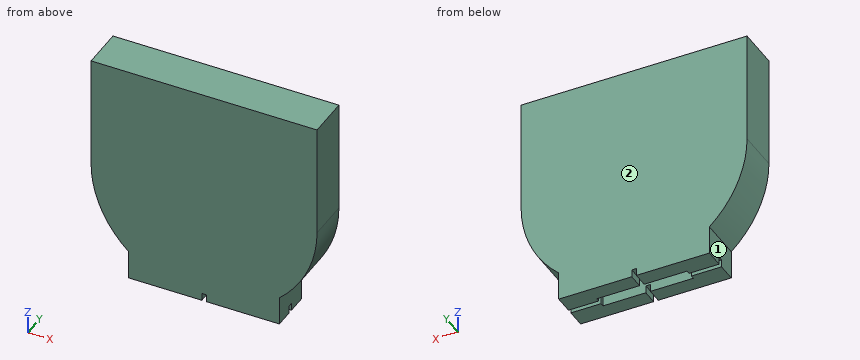
```python
from build123d import *

# Parameters (mm, degrees)
BOSS_EXTRUDE1_DEPTH = 0.8
BOSS_EXTRUDE2_DEPTH = 1
BOSS_EXTRUDE3_START = 1
BOSS_EXTRUDE3_DEPTH = 1
CUT_EXTRUDE1_DEPTH  = 0.5


with BuildPart() as part:
    # Sketch1 → Boss-Extrude1 (new body)
    with BuildSketch(Plane(origin=(0, 0, 0), x_dir=(1, 0, 0), z_dir=(0, 1, 0))):
        with BuildLine():
            Line((-5, 7.5), (-5, 5.590169944))
            ThreePointArc((-5, 5.590169944), (-6.846531969, 3.061862178), (-7.5, 0))
            Line((-7.5, 0), (-7.5, -7.5))
            Line((-7.5, -7.5), (7.5, -7.5))
            Line((7.5, -7.5), (7.5, 0))
            ThreePointArc((7.5, 0), (6.846531969, 3.061862178), (5, 5.590169944))
            Line((5, 5.590169944), (5, 7.5))
            Line((5, 7.5), (3, 7.5))
            Line((3, 7.5), (3, 5.5))
            Line((3, 5.5), (3, 5.123475383))
            ThreePointArc((3, 5.123475383), (3.101282966, 4.684946373), (3.384615385, 4.335248401))
            ThreePointArc((3.384615385, 4.335248401), (0, -5.5), (-3.384615385, 4.335248401))
            ThreePointArc((-3.384615385, 4.335248401), (-3.101282966, 4.684946373), (-3, 5.123475383))
            Line((-3, 5.123475383), (-3, 5.5))
            Line((-3, 5.5), (-3, 7.5))
            Line((-3, 7.5), (-5, 7.5))
        make_face()
    extrude(amount=BOSS_EXTRUDE1_DEPTH)

    # Sketch2 → Boss-Extrude2 (add)
    with BuildSketch(Plane(origin=(0, 0.8, 0), x_dir=(1, 0, 0), z_dir=(0, 1, 0))):
        with BuildLine():
            Line((5, 5.590169944), (5, 7.5))
            Line((5, 7.5), (3, 7.5))
            Line((3, 7.5), (-3, 7.5))
            Line((-3, 7.5), (-5, 7.5))
            Line((-5, 7.5), (-5, 5.590169944))
            ThreePointArc((-5, 5.590169944), (-6.846531969, 3.061862178), (-7.5, 0))
            Line((-7.5, 0), (-7.5, -7.5))
            Line((-7.5, -7.5), (7.5, -7.5))
            Line((7.5, -7.5), (7.5, 0))
            ThreePointArc((7.5, 0), (6.846531969, 3.061862178), (5, 5.590169944))
        make_face()
    extrude(amount=BOSS_EXTRUDE2_DEPTH)

    # Sketch3 → Boss-Extrude3 (add)
    with BuildSketch(Plane.XZ.offset(BOSS_EXTRUDE3_START)):
        with BuildLine():
            Line((-3, -7.5), (-5, -7.5))
            Line((-5, -7.5), (-5, -5.590169944))
            ThreePointArc((-5, -5.590169944), (-6.846531969, -3.061862178), (-7.5, 0))
            Line((-7.5, 0), (-7.5, 7.5))
            Line((-7.5, 7.5), (7.5, 7.5))
            Line((7.5, 7.5), (7.5, 0))
            ThreePointArc((7.5, 0), (6.846531969, -3.061862178), (5, -5.590169944))
            Line((5, -5.590169944), (5, -7.5))
            Line((5, -7.5), (3, -7.5))
            Line((3, -7.5), (-3, -7.5))
        make_face()
    extrude(amount=-BOSS_EXTRUDE3_DEPTH)

    # Sketch4 → Cut-Extrude1 (cut)
    with BuildSketch(Plane(origin=(0, 0, -7.5), x_dir=(-1, 0, 0), z_dir=(0, 0, -1))):
        Polygon((-5, 0.55), (-0.15, 0.55), (-0.15, 1.8), (0.15, 1.8), (0.15, 0.55), (5, 0.55), (5, 0.25), (0.15, 0.25), (0.15, -1), (-0.15, -1), (-0.15, 0.25), (-5, 0.25), align=None)
    extrude(amount=-CUT_EXTRUDE1_DEPTH, mode=Mode.SUBTRACT)


solid = part.part
```
The model under review builds one solid part; all positions refer to its coordinate system, in mm. Face numbers are marked on the shaded views. A direction names the side the tool comes from. Give positions to 0.01 mm unless a question says otherwise; leave off trailing zeros. Loops run counter-clockwise (first coordinate to the right, second up) from the corner with the lowest first, then second, coordinate; pieces in that order, holes last. Notation, with made-up numbers: (15.25, 89.5) - (64.25, 89.5) arc R21 cw to (64.25, 114.5) - close; hole circle Ø6 at (-23, 46). An arc over 180 degrees is marked (long way). Answer as a JSON object with one key per item and string values.
Q1. Insertion check: pin 1 (1 mm diameter, centred on y = 0.5, z = -6.5, fed in from -X). The pin has a flat end and moves straight along its axis. Give the tip position at first contact, or say it passes through.
Worked out:
{"pin 1": "stops at x = -5"}
Q2. Add section D-D on z = 3.5. State the section outline as (x, y) points.
Worked out:
{"outline": "(-7.5, -1) - (7.5, -1) - (7.5, 1.8) - (-7.5, 1.8) - close; hole (-4.24, 0) - (4.24, 0) - (4.24, 0.8) - (-4.24, 0.8) - close"}
Q3. Add section A-A on z = 0.25. State the section outline as (x, y) points, plus the area to 3 significant figures.
Worked out:
{"outline": "(-7.5, -1) - (7.5, -1) - (7.5, 1.8) - (-7.5, 1.8) - close; hole (-5.49, 0) - (5.49, 0) - (5.49, 0.8) - (-5.49, 0.8) - close", "area": "33.2 mm^2"}
Q4. Add section C-C on x = -2.25. State the section outline as (y, z) points, plus the area to 3 significant figures.
Worked out:
{"outline": "(-1, -7.5) - (0, -7.5) - (0, 5.02) - (0.8, 5.02) - (0.8, -7.5) - (1.8, -7.5) - (1.8, 7.5) - (-1, 7.5) - close", "area": "32.0 mm^2"}
Q5. To check wall thickness, follow line 1 along X through (y, z) = (0.5, 0); line 2 along Y through (x, z) = (-2, -3); line 3 along Z through (x, y) = (0, 0.2). State the ranges of each line that lie inside material, in increasing order.
Worked out:
{"line 1": "x = -7.5 to -5.5, 5.5 to 7.5", "line 2": "y = -1 to 0, 0.8 to 1.8", "line 3": "z = 5.5 to 7.5"}
Q6. For the marked faces 1 and 2, list the 3-axis set-ups (+Z, -Z, +X, -X, +Y, -Y) from which the entire face can be reached by the end or side of a thin tool; tool diameter is ignored.
Worked out:
{"face 1": "-Z, -X, +Y, -Y", "face 2": "+Z, -Z, +X, -X, +Y"}
Q7. Add section B-B on y = -0.8. State the section outline as (x, z) points, plus the area to 3 significant figures.
Worked out:
{"outline": "(-7.5, 0) arc R7.5 ccw to (-5, -5.59) - (-5, -7.5) - (-0.15, -7.5) - (-0.15, -7) - (0.15, -7) - (0.15, -7.5) - (5, -7.5) - (5, -5.59) arc R7.5 ccw to (7.5, 0) - (7.5, 7.5) - (-7.5, 7.5) - close", "area": "207 mm^2"}
